from build123d import *

# Parameters (mm, degrees)
SKETCH1_W                                           = 100
SKETCH1_H                                           = 100
BOSS_EXTRUDE1_DEPTH                                 = 10
CBORE_FOR_M6_HEX_SOCKET_HEAD_CAP_SCREW1_D           = 7
CBORE_FOR_M6_HEX_SOCKET_HEAD_CAP_SCREW1_DEPTH       = 17.946987833
CBORE_FOR_M6_HEX_SOCKET_HEAD_CAP_SCREW1_CBORE_D     = 11
CBORE_FOR_M6_HEX_SOCKET_HEAD_CAP_SCREW1_CBORE_DEPTH = 6.4
CBORE_FOR_M6_HEX_SOCKET_HEAD_CAP_SCREW1_TIP         = 2.103012167
FILLET1_R                                           = 5
SKETCH4_R                                           = 1
BOSS_EXTRUDE2_DEPTH                                 = 3.2
SKETCH5_R                                           = 2.5
BOSS_EXTRUDE3_DEPTH                                 = 2
CUT_EXTRUDE1_START                                  = -3
CUT_EXTRUDE1_DEPTH                                  = 3
LPATTERN1_COUNT                                     = 2
LPATTERN1_PITCH                                     = 87.5
LPATTERN1_COUNT_DIR2                                = 2
LPATTERN1_PITCH_DIR2                                = 87.5


with BuildPart() as part:
    # Sketch1 → Boss-Extrude1 (new body)
    with BuildSketch(Plane(origin=(0, 0, 0), x_dir=(1, 0, 0), z_dir=(0, 1, 0))):
        Rectangle(SKETCH1_W, SKETCH1_H)
    extrude(amount=BOSS_EXTRUDE1_DEPTH)

    # CBORE for M6 Hex Socket Head Cap Screw1
    with Locations(Plane(origin=(0, 10, 0), x_dir=(1, 0, 0), z_dir=(0, 1, 0))):
        with Locations((-37.5, -37.5), (37.5, -37.5), (37.5, 37.5), (-37.5, 37.5)):
            CounterBoreHole(CBORE_FOR_M6_HEX_SOCKET_HEAD_CAP_SCREW1_D / 2, CBORE_FOR_M6_HEX_SOCKET_HEAD_CAP_SCREW1_CBORE_D / 2, CBORE_FOR_M6_HEX_SOCKET_HEAD_CAP_SCREW1_CBORE_DEPTH, depth=CBORE_FOR_M6_HEX_SOCKET_HEAD_CAP_SCREW1_DEPTH)
            with Locations((0, 0, -(CBORE_FOR_M6_HEX_SOCKET_HEAD_CAP_SCREW1_DEPTH + CBORE_FOR_M6_HEX_SOCKET_HEAD_CAP_SCREW1_TIP / 2))):  # 118° drill point
                Cone(0, CBORE_FOR_M6_HEX_SOCKET_HEAD_CAP_SCREW1_D / 2, CBORE_FOR_M6_HEX_SOCKET_HEAD_CAP_SCREW1_TIP, mode=Mode.SUBTRACT)

    # Fillet1
    fillet1_edges = [part.edges().sort_by_distance(p)[0] for p in [
        (50, 5, 50),
        (-50, 5, 50),
        (-50, 5, -50),
        (50, 5, -50),
    ]]
    fillet(fillet1_edges, radius=FILLET1_R)

    # Sketch4 → Boss-Extrude2 (add)
    with BuildSketch(Plane(origin=(0, 10, 0), x_dir=(1, 0, 0), z_dir=(0, 1, 0))):
        with Locations(Location((-43.75, 43.75, 0), (0, 0, 270))):
            Circle(SKETCH4_R)
        with Locations(Location((43.75, 43.75, 0), (0, 0, 270))):
            Circle(SKETCH4_R)
        with Locations(Location((-43.75, -43.75, 0), (0, 0, 270))):
            Circle(SKETCH4_R)
        with Locations(Location((43.75, -43.75, 0), (0, 0, 270))):
            Circle(SKETCH4_R)
    extrude(amount=BOSS_EXTRUDE2_DEPTH)

    # Sketch5 → Boss-Extrude3 (add)
    with BuildSketch(Plane(origin=(0, 13.2, 0), x_dir=(1, 0, 0), z_dir=(0, 1, 0))):
        with Locations(Location((-43.75, 43.75, 0), (0, 0, 270))):
            Circle(SKETCH5_R)
        with Locations(Location((43.75, 43.75, 0), (0, 0, 270))):
            Circle(SKETCH5_R)
        with Locations(Location((43.75, -43.75, 0), (0, 0, 270))):
            Circle(SKETCH5_R)
        with Locations(Location((-43.75, -43.75, 0), (0, 0, 270))):
            Circle(SKETCH5_R)
    extrude(amount=BOSS_EXTRUDE3_DEPTH)

    # Sketch6 → Cut-Extrude1 (cut)
    with BuildSketch(Plane(origin=(0, 15.2, 0), x_dir=(1, 0, 0), z_dir=(0, 1, 0)).offset(CUT_EXTRUDE1_START)):
        with BuildLine():
            ThreePointArc((-44.75, 46.041287847), (-46.25, 43.75), (-44.75, 41.458712153))
            Line((-44.75, 41.458712153), (-44.75, 46.041287847))
        make_face()
        with BuildLine():
            Line((-42.75, 46.041287847), (-42.75, 41.458712153))
            ThreePointArc((-42.75, 41.458712153), (-41.658349934, 42.380693606), (-41.25, 43.75))
            ThreePointArc((-41.25, 43.75), (-41.658349934, 45.119306394), (-42.75, 46.041287847))
        make_face()
    cut_extrude1 = extrude(amount=CUT_EXTRUDE1_DEPTH, mode=Mode.SUBTRACT)

    # LPattern1: Cut-Extrude1 2 × 2
    with Locations(*[(j * LPATTERN1_PITCH_DIR2, 0, i * LPATTERN1_PITCH) for i in range(LPATTERN1_COUNT) for j in range(LPATTERN1_COUNT_DIR2) if (i, j) != (0, 0)]):
        add(cut_extrude1, mode=Mode.SUBTRACT)


solid = part.part
Check sheet for the modelled part. Datum: model origin and axes. Units: mm. A direction names the side the tool comes from. Round coordinates to 2 decimals unless told otherwise and drop trailing zeros. Loops run counter-clockwise (first coordinate to the right, second up) from the corner with the lowest first, then second, coordinate; pieces in that order, holes last.
1. Sectioned sample at A-A on x = 37.5. Record the boundary of the cut face in (y, z), and give its area (3 significant figures).
2. Sectioned sample at C-C on y = 1.5. Record the boundary of the cut face in (x, z).
3. Set-up check for faces 1 (the flat face through (-1, 5, 50)), 2 (the flat face through (41, 3.6, 39)): record each of +Z, -Z, +X, -X, +Y, -Y from which the full face is reachable in a straight line by a thin tool's end or side.
4. Sectioned sample at B-B on z = 37.5. Record the boundary of the cut face in (x, y).
5. Sectioned sample at D-D on y = 7. Record the boundary of the cut face in (x, z).
6. Mould release check, pull along X, two halves, no side actions. Record for faces 3 (the flat face through (-1, 5, -50)), 4 (the cylindrical face through (-42.995, 6.845, -37.742)), 5 (the flat face through (-34, 3.6, -36)), 6 (the cylindrical face through (48, 5, -49)): released by +X, released by -X, zero draft, split by the parting line, or undercut.
7. Scan lines: probe 1 along Z at (x, y) = (37.5, 6.75); probe 2 along Z at (x, y) = (-37.5, 2.55). Record each from-to range of solid material in increasing order.
8. Gauge pin test, flat ends, axial feed: pin 1 Ø2 at (y, z) = (14, -45) entering from +X; pin 2 Ø1.6 at (x, z) = (43.5, -45.5) entering from -Y; pin 3 Ø5.5 at (x, z) = (37.5, -37.5) entering from +Y; pin 4 Ø3.5 at (x, z) = (-37.5, 39.5) entering from +Y. Record the tip position at first contact, or that the pin passes through.
Recorded:
1. outline: (0, -50) - (10, -50) - (10, -43) - (3.6, -43) - (3.6, -41) - (0, -41) - close; (0, -34) - (3.6, -34) - (3.6, -32) - (10, -32) - (10, 32) - (3.6, 32) - (3.6, 34) - (0, 34) - close; (0, 41) - (3.6, 41) - (3.6, 43) - (10, 43) - (10, 50) - (0, 50) - close
1. area: 809 mm2
2. outline: (-50, -45) arc R5 ccw to (-45, -50) - (45, -50) arc R5 ccw to (50, -45) - (50, 45) arc R5 ccw to (45, 50) - (-45, 50) arc R5 ccw to (-50, 45) - close; hole circle Ø7 at (-37.5, -37.5); hole circle Ø7 at (-37.5, 37.5); hole circle Ø7 at (37.5, -37.5); hole circle Ø7 at (37.5, 37.5)
3. face 1: +Z, +X, -X, +Y, -Y
3. face 2: +Y
4. outline: (-50, 0) - (-41, 0) - (-41, 3.6) - (-43, 3.6) - (-43, 10) - (-50, 10) - close; (-34, 0) - (34, 0) - (34, 3.6) - (32, 3.6) - (32, 10) - (-32, 10) - (-32, 3.6) - (-34, 3.6) - close; (41, 0) - (50, 0) - (50, 10) - (43, 10) - (43, 3.6) - (41, 3.6) - close
5. outline: (-50, -45) arc R5 ccw to (-45, -50) - (45, -50) arc R5 ccw to (50, -45) - (50, 45) arc R5 ccw to (45, 50) - (-45, 50) arc R5 ccw to (-50, 45) - close; hole circle Ø11 at (-37.5, -37.5); hole circle Ø11 at (-37.5, 37.5); hole circle Ø11 at (37.5, -37.5); hole circle Ø11 at (37.5, 37.5)
6. face 3: zero draft
6. face 4: undercut
6. face 5: undercut
6. face 6: released by +X
7. probe 1: z = -50 to -43, -32 to 32, 43 to 50
7. probe 2: z = -50 to -41, -34 to 34, 41 to 50
8. pin 1: stops at x = 44.75
8. pin 2: stops at y = 0
8. pin 3: passes through
8. pin 4: stops at y = 3.6
